Check sheet for the modelled part. Datum: model origin and axes. Units: mm. Face numbers are marked on the shaded views. A direction names the side the tool comes from. Coordinates: 2 decimals unless noted, no trailing zeros. Loops run counter-clockwise (first coordinate to the right, second up) from the corner with the lowest first, then second, coordinate; pieces in that order, holes last. Notation, with made-up numbers: (-31, 81.25) - (-21, 81.25) arc R27 cw to (-21, 114.25) - close; hole circle Ø2 at (46, 62.5). An arc over 180 degrees is marked (long way). Answer as a JSON object with one key per item and string values. Group by question number.
from build123d import *

# Parameters (mm, degrees)
F0_R     = 7.615
F1_DEPTH = 8.8
F2_SIZE  = 1.5
F3_R     = 5
F4_DEPTH = 3.9
F5_R     = 5
F6_DEPTH = 3.9
F7_R     = 4.32
F8_DEPTH = 25


with BuildPart() as f1:
    # F0 (on Top) → F1 (new body)
    with BuildSketch(Plane.XY):
        Circle(F0_R)
    extrude(amount=F1_DEPTH)

    # F2
    f2_edges = [f1.edges().sort_by_distance(p)[0] for p in [
        (-7.615, 0, 8.8),
        (-7.615, 0, 0),
    ]]
    chamfer(f2_edges, length=F2_SIZE)

    # F3 (on face) → F4 (cut)
    with BuildSketch(Plane(origin=(0, 0, 0), x_dir=(1, 0, 0), z_dir=(0, 0, -1))):
        Circle(F3_R)
    extrude(amount=-F4_DEPTH, mode=Mode.SUBTRACT)

    # F5 (on face) → F6 (cut)
    with BuildSketch(Plane.XY.offset(8.8)):
        Circle(F5_R)
    extrude(amount=-F6_DEPTH, mode=Mode.SUBTRACT)

    # F7 (on face) → F8 (cut)
    with BuildSketch(Plane.XY.offset(4.9)):
        Circle(F7_R)
    extrude(amount=-F8_DEPTH, mode=Mode.SUBTRACT)


solid = f1.part
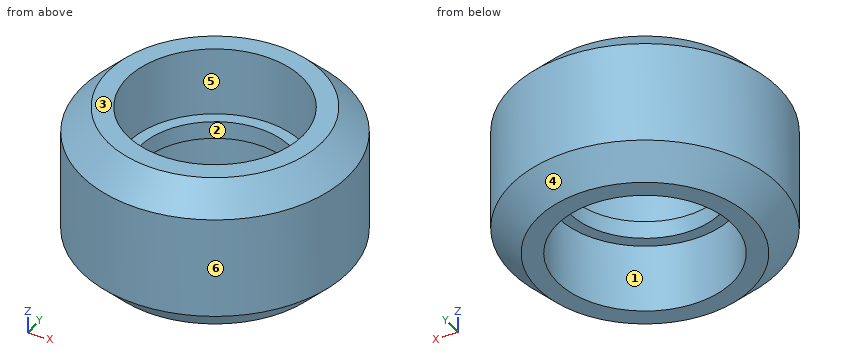
1. Sectioned sample at A-A on y = 0. Record the cut outline in (x, z) (3 decimals).
2. Sectioned sample at C-C on z = 2.25. Record the cut outline in (x, y) (3 decimals), plus the area to 3 significant figures.
3. Release check for a two-part mould opening along Y. For the marked faces 1, 2, 3 and 4 record: released by +Y, released by -Y, zero draft, split by the parting line, or undercut.
4. Gauge pin test, flat end, axial feed: pin 1 (4 mm diameter, centred on x = -6, z = 5.5, fed in from -Y). Record the tip position at first contact, or that the pin passes through.
5. Sectioned sample at D-D on z = 1.25. Record the cut outline in (x, y) (3 decimals).
6. Access from +Z, -Z, +X, -X, +Y, -Y to the whole of each face (thin tool, end or side, straight path). Record for the marked faces 5 and 6.
7. Material ranges on line 1 (Y direction, x = 0, z = 4.4) (3 decimals); line 2 (Y direction, x = 0, z = 1.65) (3 decimals); line 3 (X direction, y = -4.5, z = 8.5), recorded low to high.
Answers follow:
{
 "1": {"outline": "(-7.615, 1.5) - (-6.115, 0) - (-5, 0) - (-5, 3.9) - (-4.32, 3.9) - (-4.32, 4.9) - (-5, 4.9) - (-5, 8.8) - (-6.115, 8.8) - (-7.615, 7.3) - close; (4.32, 3.9) - (5, 3.9) - (5, 0) - (6.115, 0) - (7.615, 1.5) - (7.615, 7.3) - (6.115, 8.8) - (5, 8.8) - (5, 4.9) - (4.32, 4.9) - close"},
 "2": {"outline": "circle Ø15.23 at (0, 0); hole circle Ø10 at (0, 0)", "area": "104 mm^2"},
 "3": {"face 1": "undercut", "face 2": "undercut", "face 3": "zero draft", "face 4": "split by the parting line"},
 "4": {"pin 1": "stops at y = -6.48"},
 "5": {"outline": "circle Ø14.73 at (0, 0); hole circle Ø10 at (0, 0)"},
 "6": {"face 5": "+Z", "face 6": "+Z, -Z"},
 "7": {"line 1": "y = -7.615 to -4.32, 4.32 to 7.615", "line 2": "y = -7.615 to -5, 5 to 7.615", "line 3": "x = -4.57 to -2.18, 2.18 to 4.57"}
}
